```python
from build123d import *

# Parameters (mm, degrees)
BODY_DEPTH = 4.5
LENS_SK2_R = 3
LENS_DEPTH = 1.5


with BuildPart() as part:
    # Body_Sk1 → Body (new body)
    with BuildSketch(Plane.XY.offset(-10.2)):
        with BuildLine():
            Line((-20.31, 5.69), (-12.41, 5.69))
            ThreePointArc((-12.41, 5.69), (-12.197867966, 5.777867966), (-12.11, 5.99))
            Line((-12.11, 5.99), (-12.11, 13.89))
            ThreePointArc((-12.11, 13.89), (-12.197867966, 14.102132034), (-12.41, 14.19))
            Line((-12.41, 14.19), (-20.31, 14.19))
            ThreePointArc((-20.31, 14.19), (-20.522132034, 14.102132034), (-20.61, 13.89))
            Line((-20.61, 13.89), (-20.61, 5.99))
            ThreePointArc((-20.61, 5.99), (-20.522132034, 5.777867966), (-20.31, 5.69))
        make_face()
    extrude(amount=-BODY_DEPTH)

    # Lens_Sk2 → Lens (add)
    with BuildSketch(Plane.XY.offset(-14.7)):
        with Locations((-16.36, 9.94)):
            Circle(LENS_SK2_R)
    extrude(amount=-LENS_DEPTH)


solid = part.part
```
The listing builds one solid part. Answer for the finished solid, in the listing's coordinates (mm). A direction names the side the tool comes from. Give positions to 0.01 mm unless a question says otherwise; leave off trailing zeros. Order: outer loops, then holes, each group sorted by start corner. A loop starts at its lowest first (then second) coordinate and runs counter-clockwise, first axis right, second up.
1) Find section A-A on x = -16.36. Write down the section's boundary in (y, z).
Reported:
outline: (5.69, -14.7) - (6.94, -14.7) - (6.94, -16.2) - (12.94, -16.2) - (12.94, -14.7) - (14.19, -14.7) - (14.19, -10.2) - (5.69, -10.2) - close
2) For faces 1 (the face through (-18.741, 8.115, -15.439)), 2 (the face through (-20.61, 10, -12)), determine the directions among +Z, -Z, +X, -X, +Y, -Y from which every point of the face is accessible in a straight line to the end or side of a thin tool.
Reported:
face 1: -Z
face 2: +Z, -Z, -X, +Y, -Y
3) Find section B-B on y = 9.94. Write down the section's boundary in (x, z), then the cut area to 4 significant figures.
Reported:
outline: (-20.61, -14.7) - (-19.36, -14.7) - (-19.36, -16.2) - (-13.36, -16.2) - (-13.36, -14.7) - (-12.11, -14.7) - (-12.11, -10.2) - (-20.61, -10.2) - close
area: 47.25 mm2
4) Find section C-C on y = 13.5. Write down the section's boundary in (x, z), then the cut area to 4 significant figures.
Reported:
outline: (-20.61, -14.7) - (-12.11, -14.7) - (-12.11, -10.2) - (-20.61, -10.2) - close
area: 38.25 mm2
5) Find section D-D on x = -20. Write down the section's boundary in (y, z), then the cut area to 4 significant figures.
Reported:
outline: (5.69, -14.7) - (14.19, -14.7) - (14.19, -10.2) - (5.69, -10.2) - close
area: 38.25 mm2
6) Consider line 1 along Z through (x, y) = (-16.25, 6); line 2 along X through (y, z) = (8, -15.05); line 3 along Y through (x, z) = (-15.75, -15.8). Determine where each line is inside the solid, lowest interval first.
Reported:
line 1: z = -14.7 to -10.2
line 2: x = -18.65 to -14.07
line 3: y = 7 to 12.88
